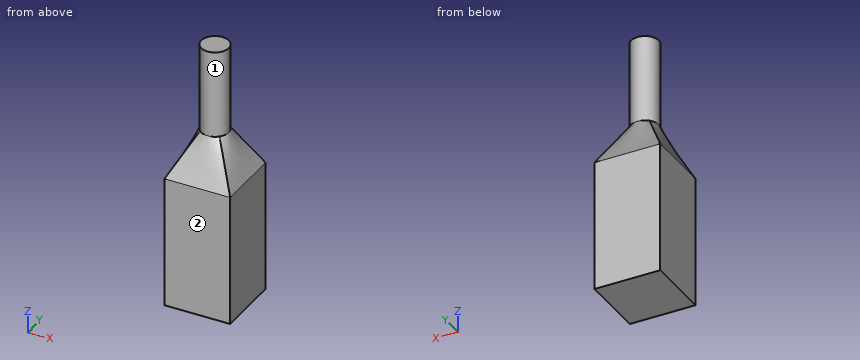
```python
from build123d import *

# Parameters (mm, degrees)
SKETCH1_W           = 19.05
SKETCH1_H           = 19.05
BOSS_EXTRUDE1_DEPTH = 38.1
SKETCH3_3_R         = 3.96875
BOSS_EXTRUDE3_DEPTH = 25.4


with BuildPart() as part:
    # Sketch1 → Boss-Extrude1 (new body)
    with BuildSketch(Plane.XY):
        with Locations((9.525, 9.525)):
            Rectangle(SKETCH1_W, SKETCH1_H)
    extrude(amount=BOSS_EXTRUDE1_DEPTH)

    # Loft3: read off the stored shape, not the designer's step
    # Loft3: loft between two sections, ruled curve by curve
    loft3_from = [
        Edge.make_bspline([(12.331330038, 12.331330038, 50.8), (12.662059205, 12.000600871, 50.8), (12.958598179, 11.583509037, 50.8), (13.375977978, 10.619086159, 50.8), (13.49375, 10.072970025, 50.8), (13.49375, 8.977029975, 50.8), (13.375977978, 8.430913841, 50.8), (12.958598179, 7.466490963, 50.8), (12.662059205, 7.049399129, 50.8), (12.331330038, 6.718669962, 50.8)], [0, 0, 0, 0, 0.25, 0.25, 0.5, 0.5, 0.75, 0.75, 1, 1, 1, 1], 3),
        Edge.make_bspline([(12.331330038, 6.718669962, 50.8), (12.000600871, 6.387940795, 50.8), (11.583509037, 6.091401821, 50.8), (10.619086159, 5.674022022, 50.8), (10.072970025, 5.55625, 50.8), (8.977029975, 5.55625, 50.8), (8.430913841, 5.674022022, 50.8), (7.466490963, 6.091401821, 50.8), (7.049399129, 6.387940795, 50.8), (6.718669962, 6.718669962, 50.8)], [0, 0, 0, 0, 0.25, 0.25, 0.5, 0.5, 0.75, 0.75, 1, 1, 1, 1], 3),
        Edge.make_bspline([(6.718669962, 12.331330038, 50.8), (7.049399129, 12.662059205, 50.8), (7.466490963, 12.958598179, 50.8), (8.430913841, 13.375977978, 50.8), (8.977029975, 13.49375, 50.8), (10.072970025, 13.49375, 50.8), (10.619086159, 13.375977978, 50.8), (11.583509037, 12.958598179, 50.8), (12.000600871, 12.662059205, 50.8), (12.331330038, 12.331330038, 50.8)], [0, 0, 0, 0, 0.25, 0.25, 0.5, 0.5, 0.75, 0.75, 1, 1, 1, 1], 3),
        Edge.make_bspline([(6.718669962, 6.718669962, 50.8), (6.387940795, 7.049399129, 50.8), (6.091401821, 7.466490963, 50.8), (5.674022022, 8.430913841, 50.8), (5.55625, 8.977029975, 50.8), (5.55625, 10.072970025, 50.8), (5.674022022, 10.619086159, 50.8), (6.091401821, 11.583509037, 50.8), (6.387940795, 12.000600871, 50.8), (6.718669962, 12.331330038, 50.8)], [0, 0, 0, 0, 0.25, 0.25, 0.5, 0.5, 0.75, 0.75, 1, 1, 1, 1], 3),
    ]
    loft3_to = [
        Edge.make_bspline([(19.05, 19.05, 38.1), (19.05, 17.4625, 38.1), (19.05, 15.875, 38.1), (19.05, 12.7, 38.1), (19.05, 11.1125, 38.1), (19.05, 7.9375, 38.1), (19.05, 6.35, 38.1), (19.05, 3.175, 38.1), (19.05, 1.5875, 38.1), (19.05, 0, 38.1)], [0, 0, 0, 0, 0.25, 0.25, 0.5, 0.5, 0.75, 0.75, 1, 1, 1, 1], 3),
        Edge.make_bspline([(19.05, 0, 38.1), (17.4625, 0, 38.1), (15.875, 0, 38.1), (12.7, 0, 38.1), (11.1125, 0, 38.1), (7.9375, 0, 38.1), (6.35, 0, 38.1), (3.175, 0, 38.1), (1.5875, 0, 38.1), (0, 0, 38.1)], [0, 0, 0, 0, 0.25, 0.25, 0.5, 0.5, 0.75, 0.75, 1, 1, 1, 1], 3),
        Edge.make_bspline([(0, 19.05, 38.1), (1.5875, 19.05, 38.1), (3.175, 19.05, 38.1), (6.35, 19.05, 38.1), (7.9375, 19.05, 38.1), (11.1125, 19.05, 38.1), (12.7, 19.05, 38.1), (15.875, 19.05, 38.1), (17.4625, 19.05, 38.1), (19.05, 19.05, 38.1)], [0, 0, 0, 0, 0.25, 0.25, 0.5, 0.5, 0.75, 0.75, 1, 1, 1, 1], 3),
        Edge.make_bspline([(0, 0, 38.1), (0, 1.5875, 38.1), (0, 3.175, 38.1), (0, 6.35, 38.1), (0, 7.9375, 38.1), (0, 11.1125, 38.1), (0, 12.7, 38.1), (0, 15.875, 38.1), (0, 17.4625, 38.1), (0, 19.05, 38.1)], [0, 0, 0, 0, 0.25, 0.25, 0.5, 0.5, 0.75, 0.75, 1, 1, 1, 1], 3),
    ]
    loft3 = Solid(Shell([*[Face.make_surface_from_curves(loft3_from[k], loft3_to[k]) for k in range(4)], Face(Wire(loft3_from)), Face(Wire(loft3_to))]))
    add(loft3)

    # Sketch3<3> → Boss-Extrude3 (add)
    with BuildSketch(Plane.XY.offset(50.8)):
        with Locations(Location((9.525, 9.525, 0), (0, 0, 135))):
            Circle(SKETCH3_3_R)
    extrude(amount=BOSS_EXTRUDE3_DEPTH)


solid = part.part
```
The listing builds one solid part. Answer for the finished solid, in the listing's coordinates (mm). Face numbers are marked on the shaded views. A direction names the side the tool comes from. Give positions to 0.01 mm unless a question says otherwise; leave off trailing zeros. Loops run counter-clockwise (first coordinate to the right, second up) from the corner with the lowest first, then second, coordinate; pieces in that order, holes last. Notation, with made-up numbers: M 88,3.5 L 126,3.5 A21 cw 126,21.5 Z; hole C 43,-22 d5. An arc over 180 degrees is marked long. One line per item, written item: value.
Q1. Flat-ended cylindrical pins translate along their axes: P1, Ø1.5, axis at x = 3.5, y = 16.5, coming from the +Z side; P2, Ø1.5, axis at x = 5, y = 5, coming from the +Z side; P3, Ø3, axis at x = 5.5, z = 57, coming from the -Y side; P4, Ø10, axis at x = 4, z = 32, coming from the -Y side. Find the tip coordinate at first contact, or state that the pin passes through.
Working result:
P1: stops at z = 44.41
P2: stops at z = 48.55
P3: stops at y = 6.46
P4: stops at y = 0
Q2. A cutting plane is placed at A-A on z = 53.5. Determine the outline of the cut face in (x, y) (1 decimal), then the cut area to 3 significant figures.
Working result:
outline: C 9.5,9.5 d7.9
area: 49.5 mm^2
Q3. Find the intervals of material crossed by line 1 (Z direction, x = 16.75, y = 14.5); line 2 (X direction, y = 13, z = 65); line 3 (Y direction, x = 8, z = 41), in increasing order. Write a range as from..to.
Working result:
line 1: z = 0..42.83
line 2: x = 7.61..11.44
line 3: y = 1.28..17.77
Q4. For the marked faces 1 and 2, determine the directions among +Z, -Z, +X, -X, +Y, -Y from which every point of the face is accessible in a straight line to the end or side of a thin tool.
Working result:
face 1: +Z
face 2: +Z, -Z, +X, -X, -Y
